Source: three-view drawing plus pictorial views. Frame: mm from the lowest corner of the part. Round coordinates to 2 decimals unless told otherwise and drop trailing zeros. Order: outer loops, then holes, each group sorted by start corner. A loop starts at its lowest first (then second) coordinate and runs counter-clockwise, first axis right, second up. Notation, with made-up numbers: (37.5, 31) -> (45.5, 31) arc R29 cw to (45.5, 51) -> close; hole circle Ø10 at (83.25, 21.25). An arc over 180 degrees is marked (long way). Answer as CSV lines item,"result". Start each with the question number.
1) Section query A-A, the plane y = 36.5. Output: boundary loops of the cut face in (x, z).
2) Line query: L1, parallel to X at y = 6, z = 36.5; L2, parallel to Y at x = 31, z = 33; L3, parallel to Y at x = 84, z = 17. Output: solid intervals per line, ascending.
3) Section query D-D, the plane y = 69. Output: boundary loops of the cut face in (x, z).
4) First-contact query: P1, Ø12, axis at x = 21.5, z = 65, coming from the +Y side; P2, Ø1.5, axis at x = 58, y = 62.5, coming from the +Z side; P3, Ø3, axis at y = 23, z = 36, coming from the -X side. Flat tips, straight axial feed; report the tip coordinate or a pass-through.
5) Section query C-C, the plane x = 43. Output: boundary loops of the cut face in (y, z).
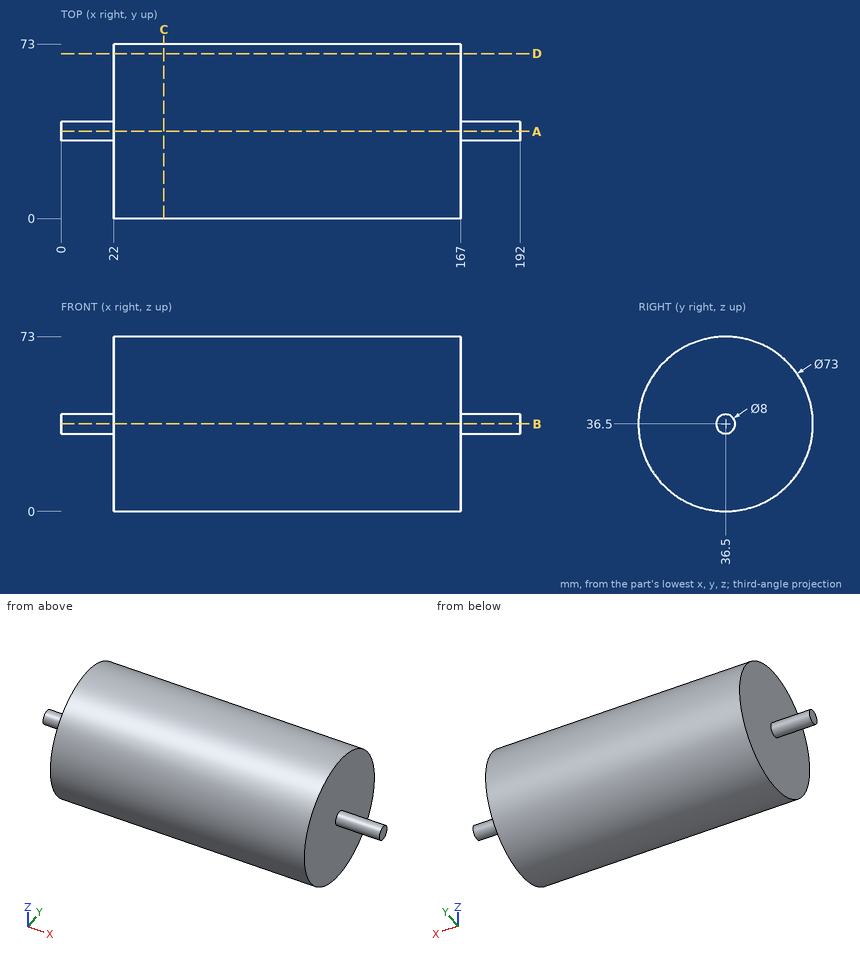
Findings:
1,outline,"(0, 32.5) -> (22, 32.5) -> (22, 0) -> (167, 0) -> (167, 32.5) -> (192, 32.5) -> (192, 40.5) -> (167, 40.5) -> (167, 73) -> (22, 73) -> (22, 40.5) -> (0, 40.5) -> close"
2,L1,"x = 22 to 167"
2,L2,"y = 0.17 to 72.83"
2,L3,"y = 5.65 to 67.35"
3,outline,"(22, 19.89) -> (167, 19.89) -> (167, 53.11) -> (22, 53.11) -> close"
4,P1,"stops at y = 65.22"
4,P2,"stops at z = 62.86"
4,P3,"stops at x = 22"
5,outline,"circle Ø73 at (36.5, 36.5)"
